The listing builds one solid part. Answer for the finished solid, in the listing's coordinates (mm). Coordinates: 2 decimals unless noted, no trailing zeros. Write each loop counter-clockwise with the first axis right and the second up, starting at its lowest first coordinate (ties: lowest second). Pieces come first, ordered by that corner, then holes.
(1) The part is cut by section A-A on z = -90. Determine the outline of the cut face in (x, y).
(2) Straight lines are drawn through the part: line 1 (Y direction, x = 2.9, z = -90); line 2 (Z direction, x = 4.65, y = -81); line 3 (Y direction, x = 5.6, z = -64). For each, find the intervals that lie inside material, in ascending order.
(3) Given P1, Ø3, axis at x = 4, z = -60, coming from the -Y side; P2, Ø8, axis at y = -20, z = -18, coming from the -X side; P3, Ø5, axis at y = -80, z = -90, coming from the +X side, each flat-ended and moving along its own axis, determine where each tip first touches the part or whether it passes through.
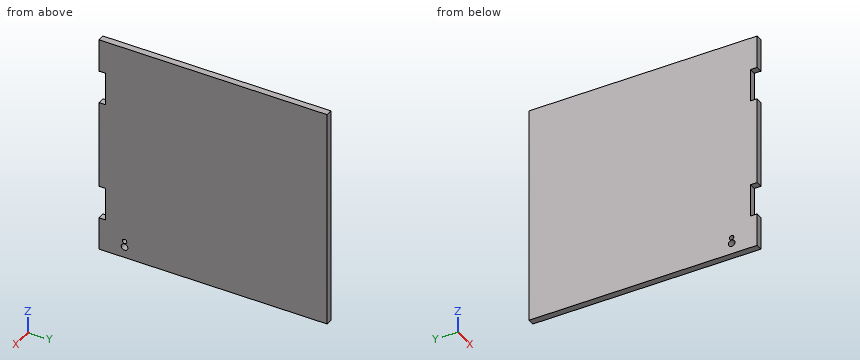
from build123d import *

# Parameters (mm, degrees)
RESSALTO_EXTRUS_O3_DEPTH = 6
ESBO_O3_R                = 3
ESBO_O3_R_2              = 2
CORTE_EXTRUS_O4_DEPTH    = 6


with BuildPart() as part:
    # Esboço1 → Ressalto-extrusão3 (new body)
    with BuildSketch(Plane(origin=(0, 0, 0), x_dir=(0, 0, -1), z_dir=(1, 0, 0))):
        Polygon((-70, -103), (-100, -103), (-100, 103), (100, 103), (100, -103), (70, -103), (70, -97), (40, -97), (40, -103), (-40, -103), (-40, -97), (-70, -97), align=None)
    extrude(amount=RESSALTO_EXTRUS_O3_DEPTH)

    # Esboço3 → Corte-extrusão4 (cut)
    with BuildSketch(Plane(origin=(6, 0, 0), x_dir=(0, 0, -1), z_dir=(1, 0, 0))):
        with Locations((90, -80)):
            Circle(ESBO_O3_R)
        with Locations((84.7, -80)):
            Circle(ESBO_O3_R_2)
    extrude(amount=-CORTE_EXTRUS_O4_DEPTH, mode=Mode.SUBTRACT)


solid = part.part
Model answer:
1. outline: (0, -103) - (6, -103) - (6, -83) - (0, -83) - close; (0, -77) - (6, -77) - (6, 103) - (0, 103) - close
2. line 1: y = -103 to -83, -77 to 103
2. line 2: z = -100 to -92.83, -87.17 to -86.43, -82.97 to 100
2. line 3: y = -97 to 103
3. P1: stops at y = -97
3. P2: stops at x = 0
3. P3: passes through
